from build123d import *

# Parameters (mm, degrees)
F0_W     = 224
F0_H     = 94
F1_DEPTH = 157
F2_R     = 10
F3_R     = 10
F5_R     = 30
F6_DEPTH = 30


with BuildPart() as f1:
    # F0 (on Front) → F1 (new body, symmetric)
    with BuildSketch(Plane.XZ):
        Rectangle(F0_W, F0_H)
    extrude(amount=F1_DEPTH, both=True)

    # F2
    f2_edges = [f1.edges().sort_by_distance(p)[0] for p in [
        (-112, -157, 0),
        (0, -157, -47),
        (112, -157, 0),
        (0, -157, 47),
    ]]
    fillet(f2_edges, radius=F2_R)

    # F3
    f3_edges = [f1.edges().sort_by_distance(p)[0] for p in [
        (-112, 157, 0),
        (0, 157, -47),
        (112, 157, 0),
        (0, 157, 47),
    ]]
    fillet(f3_edges, radius=F3_R)

    # F5 (on offset) → F6 (cut)
    with BuildSketch(Plane.YZ.offset(82)):
        Circle(F5_R)
    extrude(amount=F6_DEPTH, mode=Mode.SUBTRACT)


solid = f1.part
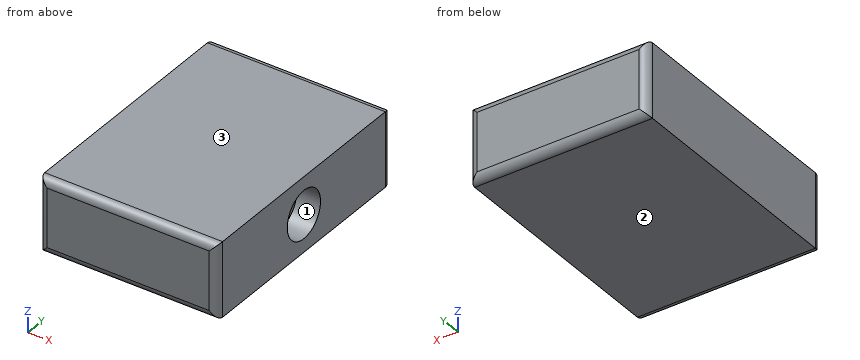
Here's how the part is built. I have some questions about the finished solid (model axes, mm). Face numbers are marked on the shaded views. Round coordinates to 2 decimals unless told otherwise and drop trailing zeros. Loops run counter-clockwise (first coordinate to the right, second up) from the corner with the lowest first, then second, coordinate; pieces in that order, holes last. Notation, with made-up numbers: M -17.5,82 L 13.5,82 A11 ccw 13.5,87 Z; hole C 21.25,52 d11. An arc over 180 degrees is marked long. Write each question's results on one line, items separated by ' | '. Start each with the question number.
(1) If I drill on probe 1 along Z at (x, y) = (100, 0); probe 2 along X at (y, z) = (-6, -14); probe 3 along Y at (x, z) = (20, 43), over which ranges is the centre line in solid material (lowest first)? Write a range as from..to.
(2) I want a section at B-B (z = 0). Please give me the cut outline in (x, y).
(3) Thinking about a two-plate mould opening in Z: for the marked faces 1, 2 and 3, which applies, pulls with the +Z half, pulls with the -Z half, needs draft (parallel to the pull), parting line crosses it, or undercut?
(4) I want a section at C-C (z = 14). Please give me the cut outline in (x, y).
(5) I want a section at A-A (y = 0). Please give me the cut outline in (x, z), then the cut area to 3 significant figures.
Solved:
1) probe 1: z = -47..-30, 30..47 | probe 2: x = -112..82 | probe 3: y = -155..155
2) outline: M -112,-147 A10 ccw -102,-157 L 102,-157 A10 ccw 112,-147 L 112,-30 L 82,-30 L 82,30 L 112,30 L 112,147 A10 ccw 102,157 L -102,157 A10 ccw -112,147 Z
3) face 1: undercut | face 2: pulls with the -Z half | face 3: pulls with the +Z half
4) outline: M -112,-147 A10 ccw -102,-157 L 102,-157 A10 ccw 112,-147 L 112,-26.53 L 82,-26.53 L 82,26.53 L 112,26.53 L 112,147 A10 ccw 102,157 L -102,157 A10 ccw -112,147 Z
5) outline: M -112,-47 L 112,-47 L 112,-30 L 82,-30 L 82,30 L 112,30 L 112,47 L -112,47 Z | area: 19,300 mm²
